Autodesk Inventor part; units mm, degrees
ref_plane "YZ Plane" through (0, 0, 0) normal (1, 0, 0) x (0, 1, 0)
ref_plane "XZ Plane" through (0, 0, 0) normal (0, 1, 0) x (-1, 0, 0)
ref_plane "XY Plane" through (0, 0, 0) normal (0, 0, 1) x (1, 0, 0)
sketch "Sketch1" plane through (0, 0, 0) normal (0, 1, 0) x (-1, 0, 0)
  circle A0 centre (0, 0) radius 7
  dimension "d0" = 14
extrude "Extrusion1" add sketch "Sketch1" along normal blind 5
sketch "Sketch2" plane through (0, 5, 0) normal (0, 1, 0) x (1, 0, 0)
  circle A0 centre (0, 0) radius 4
  dimension "d3" = 8
extrude "Extrusion2" cut sketch "Sketch2" against normal blind 3
sketch "Sketch3" plane through (0, 2, 0) normal (0, 1, 0) x (1, 0, 0)
  circle A0 centre (0, 0) radius 2
  dimension "d6" = 4
extrude "Extrusion3" cut sketch "Sketch3" against normal through all
sketch "Sketch4" plane through (0, 0, 0) normal (0, -1, 0) x (1, 0, 0)
  circle A0 centre (0, 0) radius 10
  circle A1 centre (0, 0) radius 7
  dimension "d9" = 20
extrude "Extrusion4" add sketch "Sketch4" against normal blind 2
chamfer "Chamfer1" distance 2 angle 45 1 edges at (-10, 2, 0)
properties part number "spacer_short"
Read the model definition and answer for the solid it produces. Units are mm, in the model's axes. A direction names the side the tool comes from. Give positions to 0.01 mm unless a question says otherwise; leave off trailing zeros. Write each loop counter-clockwise with the first axis right and the second up, starting at its lowest first coordinate (ties: lowest second). Pieces come first, ordered by that corner, then holes. Notation, with made-up numbers: (-15.75, 16) -> (-1.75, 16) arc R18 cw to (-1.75, 45) -> close; hole circle Ø4 at (8, -16.75). An arc over 180 degrees is marked (long way). Answer in a Markdown table with one row per item.
1) Section D-D on y = 1 is taken. Give the vertices of the cut face in (x, z), plus the area to 3 significant figures.
Results list:
| item | result |
|---|---|
| outline | circle Ø18 at (0, 0); hole circle Ø4 at (0, 0) |
| area | 242 mm^2 |
2) A tool of negligible diameter and unlimited length cuts with its end or side. For faces 4 (the cylindrical face through (0, 1, 2)), 5 (the cylindrical face through (-0.867, 3.521, 3.905)), from which of +Z, -Z, +X, -X, +Y, -Y can it reach the whole face along a straight path? Write none if from no direction.
Results list:
| item | result |
|---|---|
| face 4 | +Y, -Y |
| face 5 | +Y |
3) Each of these flat-tipped pins is pushed along its axis until it touches: pin 1 Ø4 at (x, z) = (0.5, 0) entering from +Y; pin 2 Ø1.5 at (y, z) = (1.5, 0) entering from -X; pin 3 Ø1.5 at (x, y) = (-4.5, 2.5) entering from -Z. Where does it stop, or does it pass through?
Results list:
| item | result |
|---|---|
| pin 1 | y = 2 |
| pin 2 | x = -9.25 |
| pin 3 | z = -7.03 |
4) Section C-C on y = 3.15 is taken. Give the vertices of the cut face in (x, z), plus the area to 3 significant figures.
Results list:
| item | result |
|---|---|
| outline | circle Ø14 at (0, 0); hole circle Ø8 at (0, 0) |
| area | 104 mm^2 |
5) Determine the mould class of faces 1 (the cylindrical face through (-6.466, 3.479, 2.681)), 2 (the flat face through (-2, 2, 1)), 3 (the flat face through (-0.1, 0, 2.4)) for opening direction Z: released by +Z, released by -Z, zero draft, split by the parting line, or undercut.
Results list:
| item | result |
|---|---|
| face 1 | split by the parting line |
| face 2 | undercut |
| face 3 | zero draft |
6) Straight lines are drawn through the part: line 1 (Z direction, x = 0, y = 3.35); line 2 (Z direction, x = -1, y = 1.2). For each, find the intervals that lie inside material, in ascending order. Write a range as [from, to].
Results list:
| item | result |
|---|---|
| line 1 | [-7, -4], [4, 7] |
| line 2 | [-8.74, -1.73], [1.73, 8.74] |
